CAD build for the part. Positions are in the model's coordinates, mm. A direction names the side the tool comes from. Round coordinates to 2 decimals unless told otherwise and drop trailing zeros. Loops run counter-clockwise (first coordinate to the right, second up) from the corner with the lowest first, then second, coordinate; pieces in that order, holes last.
from build123d import *

# Parameters (mm, degrees)
BOSS_EXTRUDE1_DEPTH = 21.4376
CUT_EXTRUDE1_DEPTH  = 22.4376
CUT_EXTRUDE2_DEPTH  = 2.5748
CUT_EXTRUDE3_DEPTH  = 24.107195496
CUT_EXTRUDE4_DEPTH  = 2.5748
CUT_EXTRUDE5_DEPTH  = 24.106279195
CHAMFER1_SIZE       = 1.6256
FILLET1_R           = 0.8128
FILLET2_R           = 2.3876


with BuildPart() as part:
    # Sketch1 → Boss-Extrude1 (new body)
    with BuildSketch(Plane(origin=(10.7188, 0, 0), x_dir=(0, 0, -1), z_dir=(1, 0, 0))):
        Polygon((-23.106279195, 17.785895496), (-23.106279195, -5.3213), (0, -5.3213), (0, 6.310276302), (-11.475619195, 17.785895496), align=None)
    extrude(amount=-BOSS_EXTRUDE1_DEPTH)

    # Sketch2 → Cut-Extrude1 (cut, through all)
    with BuildSketch(Plane.ZY.offset(10.7188)):
        Polygon((23.106279195, -5.3213), (23.106279195, 16.211095496), (12.127922713, 16.211095496), (1.5748, 5.657972783), (1.5748, -5.3213), align=None)
    extrude(amount=-CUT_EXTRUDE1_DEPTH, mode=Mode.SUBTRACT)

    # Sketch3 → Cut-Extrude2 (cut, through all)
    with BuildSketch(Plane.XZ.offset(-16.211095496)):
        with BuildLine():
            Line((-4.2545, 17.272), (-4.2545, 19.05))
            ThreePointArc((-4.2545, 19.05), (-6.35, 21.1455), (-8.4455, 19.05))
            Line((-8.4455, 19.05), (-8.4455, 17.272))
            ThreePointArc((-8.4455, 17.272), (-6.35, 15.1765), (-4.2545, 17.272))
        make_face()
    extrude(amount=-CUT_EXTRUDE2_DEPTH, mode=Mode.SUBTRACT)

    # Sketch4 → Cut-Extrude3 (cut, through all)
    with BuildSketch(Plane(origin=(0, 17.785895496, 0), x_dir=(-1, 0, 0), z_dir=(0, 1, 0))):
        with BuildLine():
            Line((-8.4455, 19.05), (-8.4455, 17.272))
            ThreePointArc((-8.4455, 17.272), (-6.35, 15.1765), (-4.2545, 17.272))
            Line((-4.2545, 17.272), (-4.2545, 19.05))
            ThreePointArc((-4.2545, 19.05), (-6.35, 21.1455), (-8.4455, 19.05))
        make_face()
    extrude(amount=-CUT_EXTRUDE3_DEPTH, mode=Mode.SUBTRACT)

    # Sketch5 → Cut-Extrude4 (cut, through all)
    with BuildSketch(Plane.XY.offset(1.5748)):
        with BuildLine():
            Line((4.2545, 0.513895496), (4.2545, -1.264104504))
            ThreePointArc((4.2545, -1.264104504), (6.35, -3.359604504), (8.4455, -1.264104504))
            Line((8.4455, -1.264104504), (8.4455, 0.513895496))
            ThreePointArc((8.4455, 0.513895496), (6.35, 2.609395496), (4.2545, 0.513895496))
        make_face()
    extrude(amount=-CUT_EXTRUDE4_DEPTH, mode=Mode.SUBTRACT)

    # Sketch6 → Cut-Extrude5 (cut, through all)
    with BuildSketch(Plane(origin=(0, 0, 0), x_dir=(-1, 0, 0), z_dir=(0, 0, -1))):
        with BuildLine():
            Line((8.4455, -1.264104504), (8.4455, 0.513895496))
            ThreePointArc((8.4455, 0.513895496), (6.35, 2.609395496), (4.2545, 0.513895496))
            Line((4.2545, 0.513895496), (4.2545, -1.264104504))
            ThreePointArc((4.2545, -1.264104504), (6.35, -3.359604504), (8.4455, -1.264104504))
        make_face()
    extrude(amount=-CUT_EXTRUDE5_DEPTH, mode=Mode.SUBTRACT)

    # Chamfer1
    chamfer1_edges = [part.edges().sort_by_distance(p)[0] for p in [
        (10.7188, -5.3213, 0.7874),
        (-10.7188, -5.3213, 0.7874),
        (10.7188, 16.998495496, 23.106279195),
        (-10.7188, 16.998495496, 23.106279195),
    ]]
    chamfer(chamfer1_edges, length=CHAMFER1_SIZE)

    # Fillet1
    fillet1_edges = [part.edges().sort_by_distance(p)[0] for p in [
        (0, 5.657972783, 1.5748),
        (0, 16.211095496, 12.127922713),
    ]]
    fillet(fillet1_edges, radius=FILLET1_R)

    # Fillet2
    fillet2_edges = [part.edges().sort_by_distance(p)[0] for p in [
        (0, 17.785895496, 11.475619195),
        (0, 6.310276302, 0),
    ]]
    fillet(fillet2_edges, radius=FILLET2_R)


solid = part.part
Item 1: Cut at C-C (y = -2.75). List the corners of the cut face in (x, z), plus the area to 3 significant figures.
Verdict:
outline: (-10.72, 0) - (-7.83, 0) - (-7.83, 1.57) - (-10.72, 1.57) - close; (-4.87, 0) - (4.87, 0) - (4.87, 1.57) - (-4.87, 1.57) - close; (7.83, 0) - (10.72, 0) - (10.72, 1.57) - (7.83, 1.57) - close
area: 24.5 mm2
Item 2: Cut at D-D (x = -3). List the corners of the cut face in (y, z).
Verdict:
outline: (-5.32, 0) - (5.32, 0) arc R2.39 ccw to (7.01, 0.7) - (17.09, 10.78) arc R2.39 ccw to (17.79, 12.46) - (17.79, 23.11) - (16.21, 23.11) - (16.21, 12.46) arc R0.81 cw to (15.97, 11.89) - (5.9, 1.81) arc R0.81 cw to (5.32, 1.57) - (-5.32, 1.57) - close
Item 3: Cut at A-A (x = -6.35). List the corners of the cut face in (y, z).
Verdict:
outline: (-5.32, 0) - (-3.36, 0) - (-3.36, 1.57) - (-5.32, 1.57) - close; (2.61, 0) - (5.32, 0) arc R2.39 ccw to (7.01, 0.7) - (17.09, 10.78) arc R2.39 ccw to (17.79, 12.46) - (17.79, 15.18) - (16.21, 15.18) - (16.21, 12.46) arc R0.81 cw to (15.97, 11.89) - (5.9, 1.81) arc R0.81 cw to (5.32, 1.57) - (2.61, 1.57) - close; (16.21, 21.15) - (17.79, 21.15) - (17.79, 23.11) - (16.21, 23.11) - close
Item 4: Wall check: L1, parallel to Y at x = 3, z = 17.5; L2, parallel to X at y = -2, z = 1.5; L3, parallel to Z at x = 3.25, y = 3.75. Give the ranges that are in metal, low to high.
Verdict:
L1: y = 16.21 to 17.79
L2: x = -10.72 to -8.31, -4.39 to 4.39, 8.31 to 10.72
L3: z = 0 to 1.57
Item 5: Cut at B-B (z = 17.75). List the corners of the cut face in (x, y).
Verdict:
outline: (-10.72, 16.21) - (-8.45, 16.21) - (-8.45, 17.79) - (-10.72, 17.79) - close; (-4.25, 16.21) - (4.25, 16.21) - (4.25, 17.79) - (-4.25, 17.79) - close; (8.45, 16.21) - (10.72, 16.21) - (10.72, 17.79) - (8.45, 17.79) - close
Item 6: 3-axis set-ups, long thin cutter, end or side, ignore diameter. For faces 1 (the cylindrical face through (6.3, -3.36, 0.8)), 2 (the flat face through (-9.9, 17, 22.3)), 3 (the flat face through (4.254, 17, 18)): which of +Z, -Z, +X, -X, +Y, -Y reach the whole face in a straight line?
Verdict:
face 1: +Z, -Z
face 2: +Z, -X, +Y, -Y
face 3: +Y, -Y
Item 7: Flat gauge pins, fed straight in: P1, Ø5.5, axis at x = 3, y = 1.5, coming from the +Z side; P2, Ø6, axis at x = 1, z = 8, coming from the -Y side; P3, Ø8, axis at x = 4, z = 19.5, coming from the -Y side. Where does each tip first touch, or does it go through?
Verdict:
P1: stops at z = 1.57
P2: stops at y = 9.08
P3: stops at y = 16.21
Item 8: Mould opens along X. For faces 4 (the flat face through (10.719, 11.1, 6.8)), 5 (the cylindrical face through (-6.304, 16.987, 21.145)), 6 (the flat face through (0.15, 11.98, 5.67)) say: released by +X, released by -X, zero draft, split by the parting line, or undercut.
Verdict:
face 4: released by +X
face 5: undercut
face 6: zero draft
